The model under review builds one solid part; all positions refer to its coordinate system, in mm. A direction names the side the tool comes from. Coordinates: 2 decimals unless noted, no trailing zeros. Write each loop counter-clockwise with the first axis right and the second up, starting at its lowest first coordinate (ties: lowest second). Pieces come first, ordered by that corner, then holes. Notation, with made-up numbers: (74, -3) - (103, -3) arc R30 ccw to (103, 27) - close; hole circle Ø10 at (56, 59). An arc over 180 degrees is marked (long way). Put each result on its own line as item: value. Start each with the question number.
Item 1: Consider section A-A on z = 0. Give the boundary of the cut face in (x, y).
Item 2: Consider section B-B on y = 0. Give the boundary of the cut face in (x, z).
Item 3: Machinability: for faces 1 (the face through (34.784, 13.793, -3.243)), 2 (the face through (19.72, 16.992, 10.325)), 3 (the face through (19.72, -7.63, 18.29)), 4 (the face through (25.2, -2.6, 0.1)), 5 (the face through (19.72, -7.678, -18.341)), which of the approach directions +Z, -Z, +X, -X, +Y, -Y give a long, thin tool a straight path to every point of the face, cutting with its end or side? Answer none if there is none.
Item 4: Mouldability with a two-part tool opening along Y and no side actions: class faces 6 (the face through (19.72, -16.992, -10.325)), 7 (the face through (40, 5, 0)), 8 (the face through (16.544, 19.816, -1.634)) as pulls with the +Y half, pulls with the -Y half, needs draft (parallel to the pull), parting line crosses it, or undercut.
Item 5: To check wall thickness, follow L1, parallel to Z at x = 35, y = 15; L2, parallel to X at y = 14, z = 0; L3, parallel to Z at x = 9.5, y = 19.5. State the ranges of each line that lie inside material, in increasing order. Write a range as [from, to].
Item 6: For pin 1 (5 mm diameter, centred on x = 35, z = 0, fed in from -Y); pin 2 (3 mm diameter, centred on x = 35, z = 0, fed in from +Y); pin 3 (5 mm diameter, centred on x = 14.5, y = -5.5, fed in from +Z); pin 4 (1.5 mm diameter, centred on y = 17.5, z = -16.5, fed in from -X), all flat-tipped, find the tip position at first contact; note any pin that passes through.
Item 7: Consider section C-C on y = -5.5. Give the boundary of the cut face in (x, z), then the cut area to 3 significant figures.
```python
from build123d import *

# Parameters (mm, degrees)
BASPROSKE_W         = 40
BASPROSKE_H         = 22
TOOTHCUT_DEPTH      = 51.675437837
TEETHCUTS_COUNT     = 20
TEETHCUTS_ANGLE     = 342
BORSKE_R            = 0.4
BORE_DEPTH          = 50.0000508
SKETCH1_R           = 2.6
CUT_EXTRUDE1_DEPTH  = 51.50774594
BOSS_EXTRUDE1_DEPTH = 40
BOSS_EXTRUDE2_START = -10
BOSS_EXTRUDE2_DEPTH = 10
SKETCH4_R           = 3.25
CUT_EXTRUDE2_DEPTH  = 54.373293014
CUT_EXTRUDE3_REACH  = 55.373
SKETCH5_R           = 1.4


with BuildPart() as part:
    # BasProSke → Base-Revolve (revolve)
    with BuildSketch(Plane(origin=(0, 0, 0), x_dir=(1, 0, 0), z_dir=(0, 1, 0)), mode=Mode.PRIVATE) as base_revolve_sk:
        with Locations((20, 11)):
            Rectangle(BASPROSKE_W, BASPROSKE_H)
    revolve(base_revolve_sk.sketch.rotate(Axis((-10, 0, 0), (1, 0, 0)), 180), axis=Axis((-10, 0, 0), (1, 0, 0)))

    # TooCutSke → ToothCut (cut, through all)
    with BuildSketch(Plane(origin=(0, 0, 0), x_dir=(0, 0, -1), z_dir=(1, 0, 0))):
        with BuildLine():
            ThreePointArc((0.986171591, 17.471189616), (0, 17.499), (-0.986171591, 17.471189616))
            ThreePointArc((-0.986171591, 17.471189616), (-1.626916196, 19.798789858), (-2.932850173, 21.829260982))
            ThreePointArc((-2.932850173, 21.829260982), (0, 22.0254), (2.932850173, 21.829260982))
            ThreePointArc((2.932850173, 21.829260982), (1.626916196, 19.798789858), (0.986171591, 17.471189616))
        make_face()
    toothcut = extrude(amount=TOOTHCUT_DEPTH, mode=Mode.SUBTRACT)

    # TeethCuts: ToothCut ×20 about axis
    teethcuts_axis = Axis((-10, 0, 0), (1, 0, 0))
    for i in range(1, TEETHCUTS_COUNT):
        add(toothcut.rotate(teethcuts_axis, i * TEETHCUTS_ANGLE / (TEETHCUTS_COUNT - 1)), mode=Mode.SUBTRACT)

    # BorSke → Bore (cut, symmetric)
    with BuildSketch(Plane(origin=(0, 0, 0), x_dir=(0, 0, -1), z_dir=(1, 0, 0))):
        with Locations(Location((0, 0, 0), (0, 0, 180))):
            Circle(BORSKE_R)
    extrude(amount=BORE_DEPTH, both=True, mode=Mode.SUBTRACT)

    # Sketch1 → Cut-Extrude1 (cut, through all)
    with BuildSketch(Plane(origin=(40, 0, 0), x_dir=(0, 0, -1), z_dir=(1, 0, 0))):
        Circle(SKETCH1_R)
    extrude(amount=-CUT_EXTRUDE1_DEPTH, mode=Mode.SUBTRACT)

    # Sketch2 → Boss-Extrude1 (add)
    with BuildSketch(Plane.ZY):
        with BuildLine():
            Line((-2.236067977, 2), (2.236067977, 2))
            ThreePointArc((2.236067977, 2), (0, 3), (-2.236067977, 2))
        make_face()
    extrude(amount=-BOSS_EXTRUDE1_DEPTH)

    # Sketch3 → Boss-Extrude2 (add)
    with BuildSketch(Plane.ZY.offset(BOSS_EXTRUDE2_START)):
        with BuildLine():
            Line((-1.661324773, 2), (1.661324773, 2))
            ThreePointArc((1.661324773, 2), (0, -2.6), (-1.661324773, 2))
        make_face()
    extrude(amount=BOSS_EXTRUDE2_DEPTH)

    # Sketch4 → Cut-Extrude2 (cut, through all)
    with BuildSketch(Plane(origin=(0, 6, 0), x_dir=(1, 0, 0), z_dir=(0, 1, 0))):
        with Locations(Location((35, 0, 0), (0, 0, 116.335173549))):
            Circle(SKETCH4_R)
    extrude(amount=CUT_EXTRUDE2_DEPTH, mode=Mode.SUBTRACT)

    # Sketch5 → Cut-Extrude3 (cut, up to next)
    with BuildSketch(Plane(origin=(0, 6, 0), x_dir=(1, 0, 0), z_dir=(0, 1, 0)), mode=Mode.PRIVATE) as cut_extrude3_sk1:
        with Locations(Location((35, 0, 0), (0, 0, 270))):
            Circle(SKETCH5_R)
    cut_extrude3_tool1 = extrude(cut_extrude3_sk1.sketch, amount=-CUT_EXTRUDE3_REACH, mode=Mode.PRIVATE) & part.part
    add(cut_extrude3_tool1.solids().sort_by_distance((35, 6, 0))[0], mode=Mode.SUBTRACT)


solid = part.part
```
Report:
1. outline: (0, -17.5) - (40, -17.5) - (40, -2.6) - (10, -2.6) - (10, 2) - (33.6, 2) - (33.6, 6) - (31.75, 6) - (31.75, 17.5) - (0, 17.5) - close; (36.4, 2) - (40, 2) - (40, 17.5) - (38.25, 17.5) - (38.25, 6) - (36.4, 6) - close
2. outline: (0, -17.5) - (40, -17.5) - (40, -2.6) - (10, -2.6) - (10, 2.6) - (40, 2.6) - (40, 17.5) - (0, 17.5) - close
3. face 1: +Y
3. face 2: +X, -X
3. face 3: +Z, +X, -X
3. face 4: +X
3. face 5: -Z, +X, -X
4. face 6: undercut
4. face 7: needs draft
4. face 8: pulls with the +Y half
5. L1: [-15.89, -12.85], [-9.62, -3.25], [3.25, 9.62], [12.85, 15.89]
5. L2: [0, 31.75], [38.25, 40]
5. L3: [-10.19, -8.99], [-4.55, -1.5], [1.5, 4.55], [8.99, 10.19]
6. pin 1: y = -21.29
6. pin 2: y = 6
6. pin 3: z = 21.79
6. pin 4: through
7. outline: (0, -16.61) - (40, -16.61) - (40, 16.61) - (0, 16.61) - close
7. area: 1,330 mm²
